Work out the finished part from the listing and answer in its coordinate system (mm). Coordinates: 2 decimals unless noted, no trailing zeros. Order: outer loops, then holes, each group sorted by start corner. A loop starts at its lowest first (then second) coordinate and runs counter-clockwise, first axis right, second up. Notation, with made-up numbers: (38, 60) - (76, 60) arc R20 ccw to (76, 90) - close; hole circle Ø8 at (44.5, 73). An arc over 180 degrees is marked (long way). Answer as a JSON object with one key per item and string values. Group by question number.
1) Section B-B (x = -45) is taken. Give the vertices of the cut face in (y, z), plus the area to 3 significant figures.
2) Section A-A (z = 0.5) is taken. Give the vertices of the cut face in (x, y) (1 decimal).
3) Section C-C (y = 28.5) is taken. Give the vertices of the cut face in (x, z), plus the area to 3 significant figures.
4) Find the intervals of material crossed by line 1 along Y through (x, z) = (-65, 0.65); line 2 along X through (y, z) = (42.5, 0.55); line 3 along X through (y, z) = (51.5, 0.65), in increasing order.
Autodesk Inventor part; units mm, degrees
ref_plane "YZ Plane" through (0, 0, 0) normal (1, 0, 0) x (0, 1, 0)
ref_plane "XZ Plane" through (0, 0, 0) normal (0, 1, 0) x (-1, 0, 0)
ref_plane "XY Plane" through (0, 0, 0) normal (0, 0, 1) x (1, 0, 0)
sketch "スケッチ1" plane through (0, 0, 0) normal (0, 0, 1) x (1, 0, 0)
  line L0 (44.9825, 3) -> (44.9825, 0) construction
  line L1 (44.9825, 0) -> (93.5151, 0) construction
  line L2 (44.9825, 3) -> (93.5151, 3) construction
  circle A0 centre (152.1179, -73.6808) radius 5 construction
  circle A1 centre (90.7937, -5.925) radius 3 construction
  circle A2 centre (91.5613, -41.579) radius 3 construction
  line L3 (50.9825, 0) -> (47.9825, 0) construction
  line L4 (47.9825, 0.7) -> (50.9825, 0.7) construction
  circle A3 centre (110.1553, -43.629) radius 14 construction
  circle A4 centre (105.6122, -16) radius 14 construction
  arc A5 (39.4825, -0.75) -> (39.4825, -77.9308) centre (39.4825, -39.3404) ccw construction
  line L5 (-44.9825, -3) -> (-44.9825, 0)
  line L6 (-44.9825, 0) -> (-93.5151, 0)
  line L7 (-44.9825, -3) -> (-93.5151, -3)
  circle A6 centre (-152.1179, 73.6808) radius 5
  circle A7 centre (-90.7937, 5.925) radius 3
  circle A8 centre (-91.5613, 41.579) radius 3
  line L8 (-50.9825, 0) -> (-47.9825, 0)
  line L9 (-47.9825, -0.7) -> (-50.9825, -0.7)
  circle A9 centre (-110.1553, 43.629) radius 14
  circle A10 centre (-105.6122, 16) radius 14
  arc A11 (-39.4825, 0.75) -> (-39.4825, 77.9308) centre (-39.4825, 39.3404) ccw
  line L10 (-97.013, 53.9033) -> (-2.9368, 53.9033)
  circle A12 centre (-91.5613, 41.579) radius 1.5
  circle A13 centre (-90.7937, 5.925) radius 1.5
  line L11 (-97.013, 53.9033) -> (-89.1899, 13.6565)
  line L12 (-89.1899, 13.6565) -> (-98.7082, -0.429)
  line L13 (0, 0) -> (-132.2518, 0)
  line L14 (-98.4183, 0) -> (-39.4825, 0)
  arc A14 (-39.4825, 0) -> (-39.4825, 78.6808) centre (-39.4825, 39.3404) ccw
  line L15 (-39.4825, 78.6808) -> (-39.4825, 53.9033)
  line L16 (-94.9784, 43.4362) -> (-69.0084, 53.9033)
  line L17 (-92.9751, 3.8654) -> (-89.8036, 0)
  point P0 (49.4825, 0.7)
  point P1 (-49.4825, -0.7)
  point P2 (-39.4825, 0)
  point P3 (-39.4825, 78.6808)
  point P4 (-92.6828, 44.3615)
  point P5 (-94.5062, 41.0065)
  point P6 (-44.9825, 0)
  point P7 (-89.8036, 0)
  point P8 (-93.2794, 7.6047)
  dimension "d2" = 360
  dimension "d4" = 3
  dimension "d5" = 3
  dimension "d6" = 1.5
  dimension "d7" = 41
  dimension "d8" = 79
  dimension "d9" = 17
  dimension "d11" = 0.75
  dimension "d14" = 28
  dimension "d16" = 5
extrude "押し出し1" add sketch "スケッチ1" along normal blind 0.75 contours L6 L17 A7 L12 L11 A8 L16 L10 A14 L13 | L10 A11 L15 A14 | L10 L15 A11 | A7 | A8
properties part number "回路BOX側面" material "ポリプロピレン"
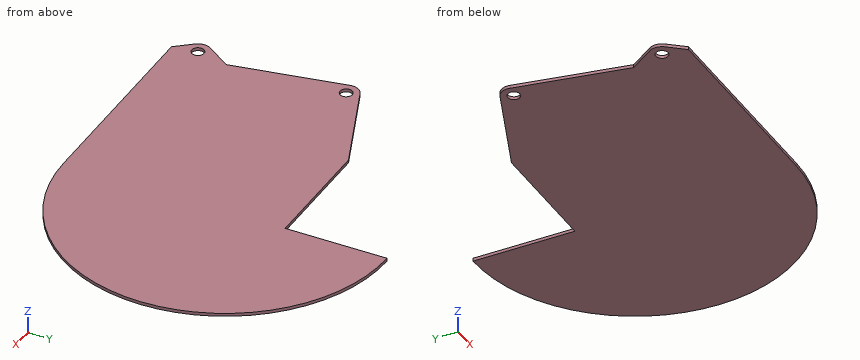
Report:
{
 "1": {"outline": "(0, 0) - (53.9, 0) - (53.9, 0.75) - (0, 0.75) - close", "area": "40.4 mm²"},
 "2": {"outline": "(-94.5, 41) - (-89.2, 13.7) - (-93.3, 7.6) arc R3 ccw to (-93, 3.9) - (-89.8, 0) - (-39.5, 0) arc R39.3 ccw to (-39.5, 78.7) - (-39.5, 53.9) - (-69, 53.9) - (-92.7, 44.4) arc R3 ccw to start; hole circle Ø3 at (-91.6, 41.6); hole circle Ø3 at (-90.8, 5.9)"},
 "3": {"outline": "(-92.08, 0) - (-1.67, 0) - (-1.67, 0.75) - (-92.08, 0.75) - close", "area": "67.8 mm²"},
 "4": {"line 1": "y = 0 to 53.9", "line 2": "x = -94.42 to -92.75, -90.38 to -0.27", "line 3": "x = -74.97 to -2.07"}
}
